from build123d import *

# Parameters (mm, degrees)
SKETCH1_R           = 4
BOSS_EXTRUDE1_DEPTH = 5
BOSS_EXTRUDE2_DEPTH = 29
FILLET1_R           = 50
FILLET2_R           = 50


with BuildPart() as part:
    # Sketch1 → Boss-Extrude1 (new body)
    with BuildSketch(Plane(origin=(0, 0, 0), x_dir=(1, 0, 0), z_dir=(0, 1, 0))):
        Polygon((-17.6, 10.161364738), (-17.6, 93), (17.6, 93), (17.6, 10.161364738), (89.340362552, -31.257952893), (71.740362552, -61.742047107), (0, -20.322729475), (-71.740362552, -61.742047107), (-89.340362552, -31.257952893), align=None)
        with Locations(Location((0, 0, 0), (0, 0, 270))):
            Circle(SKETCH1_R, mode=Mode.SUBTRACT)
        with BuildLine():
            Line((-11.5, 75), (-11.5, 71))
            ThreePointArc((-11.5, 71), (0, 59.5), (11.5, 71))
            Line((11.5, 71), (11.5, 75))
            ThreePointArc((11.5, 75), (0, 86.5), (-11.5, 75))
        make_face(mode=Mode.SUBTRACT)
        with BuildLine():
            Line((-14.875, 88), (-14.875, 84))
            ThreePointArc((-14.875, 84), (-13, 82.125), (-11.125, 84))
            Line((-11.125, 84), (-11.125, 88))
            ThreePointArc((-11.125, 88), (-13, 89.875), (-14.875, 88))
        make_face(mode=Mode.SUBTRACT)
        with BuildLine():
            Line((11.125, 88), (11.125, 84))
            ThreePointArc((11.125, 84), (13, 82.125), (14.875, 84))
            Line((14.875, 84), (14.875, 88))
            ThreePointArc((14.875, 88), (13, 89.875), (11.125, 88))
        make_face(mode=Mode.SUBTRACT)
        with BuildLine():
            Line((11.125, 62), (11.125, 58))
            ThreePointArc((11.125, 58), (13, 56.125), (14.875, 58))
            Line((14.875, 58), (14.875, 62))
            ThreePointArc((14.875, 62), (13, 63.875), (11.125, 62))
        make_face(mode=Mode.SUBTRACT)
        with BuildLine():
            Line((-14.875, 62), (-14.875, 58))
            ThreePointArc((-14.875, 58), (-13, 56.125), (-11.125, 58))
            Line((-11.125, 58), (-11.125, 62))
            ThreePointArc((-11.125, 62), (-13, 63.875), (-14.875, 62))
        make_face(mode=Mode.SUBTRACT)
    extrude(amount=BOSS_EXTRUDE1_DEPTH)

    # Sketch2 → Boss-Extrude2 (add)
    with BuildSketch(Plane.XZ):
        Polygon((-71.740362552, 61.742047107), (-89.340362552, 31.257952893), (-68.555752861, 19.257952893), (-50.955752861, 49.742047107), align=None)
        Polygon((71.740362552, 61.742047107), (89.340362552, 31.257952893), (68.555752861, 19.257952893), (50.955752861, 49.742047107), align=None)
    extrude(amount=BOSS_EXTRUDE2_DEPTH)

    # Fillet1
    # the kernel refuses this fillet: 50 mm, written as the material it adds along each edge
    with BuildSketch(Plane(origin=(-68.555752861, 0, 19.257952893), x_dir=(0, -1, 0), z_dir=(0.4999999999999999, 0, 0.8660254037844387))) as fillet1_piece_1:
        with BuildLine():
            CenterArc((50, 45.376205218), FILLET1_R, 180, 65.16541251)
            Line((0, 45.376205218), (-1, 45.376205218))
            Line((-1, 45.376205218), (-1, 0))
            Line((-1, 0), (0, -1))
            ThreePointArc((0, -1), (14.5, -1), (28.58, -0.907524104))
            Line((28.58, -0.907524104), (29, 0))
        make_face()
    extrude(amount=35.2)
    with BuildSketch(Plane(origin=(68.555752861, 0, 19.257952893), x_dir=(0, -1, 0), z_dir=(-0.49999999999999983, 0, 0.8660254037844388))) as fillet1_piece_2:
        with BuildLine():
            CenterArc((50, -45.376205218), FILLET1_R, 114.83458749, 65.16541251)
            Line((0, -45.376205218), (-1, -45.376205218))
            Line((-1, -45.376205218), (-1, 0))
            Line((-1, 0), (0, 1))
            ThreePointArc((0, 1), (14.5, 1), (28.58, 0.907524104))
            Line((28.58, 0.907524104), (29, 0))
        make_face()
    extrude(amount=35.2)
    # the kernel refuses this fillet: 50 mm, written as the material it takes off along each edge
    with BuildSketch(Plane(origin=(148.553958964, 5, -71.30300459), x_dir=(-0.8660254037844363, 0, -0.5000000000000039), z_dir=(-0.5000000000000039, 0, 0.8660254037844364)), Plane(origin=(-12.52676614, 5, 164.30300459), x_dir=(0.8660254037844429, 0, -0.4999999999999925), z_dir=(-0.49999999999999256, 0, -0.866025403784443))) as fillet1_2_piece_1:
        with BuildLine():
            CenterArc((47.370877129, 50), FILLET1_R, 198.662924885, 71.337075115)
            Line((0, 34), (-0.947417543, 33.68))
            ThreePointArc((-0.947417543, 33.68), (-1, 17), (-1, 0))
            Line((-1, 0), (0, -1))
            Line((0, -1), (47.370877129, -1))
            Line((47.370877129, -1), (47.370877129, 0))
        make_face()
    extrude(amount=272.054385647, mode=Mode.SUBTRACT)

    # Fillet2
    # the kernel refuses this fillet: 50 mm, written as the material it takes off along each edge
    with BuildSketch(Plane(origin=(-98.555752861, -29, -32.703571334), x_dir=(0.49710588531055566, 0.8188493868753551, -0.2870042166997965), z_dir=(0.4999999999999999, 0, 0.8660254037844387))) as fillet2_piece_1:
        with BuildLine():
            CenterArc((26.55146204, 49.210454923), FILLET2_R, 216.239467537, 43.564898237)
            Line((-13.776202402, 19.652385285), (-14.58275569, 19.061223892))
            ThreePointArc((-14.58275569, 19.061223892), (-7.706950588, 9.252184209), (-0.818849387, -0.574008433))
            Line((-0.818849387, -0.574008433), (0.177009747, -0.984209098))
            ThreePointArc((0.177009747, -0.984209098), (8.850487347, -0.210454923), (17.523964946, -0.984209098))
            Line((17.523964946, -0.984209098), (17.700974693, 0))
        make_face()
    extrude(amount=155.2, mode=Mode.SUBTRACT)
    with BuildSketch(Plane(origin=(98.555752861, -29, -32.703571334), x_dir=(-0.4971058853105562, 0.8188493868753546, -0.2870042166997967), z_dir=(-0.49999999999999983, 0, 0.8660254037844388))) as fillet2_piece_2:
        with BuildLine():
            CenterArc((26.55146204, -49.210454923), FILLET2_R, 100.195634226, 43.564898237)
            Line((-13.776202402, -19.652385285), (-14.58275569, -19.061223892))
            ThreePointArc((-14.58275569, -19.061223892), (-7.706950588, -9.252184209), (-0.818849387, 0.574008433))
            Line((-0.818849387, 0.574008433), (0.177009747, 0.984209098))
            ThreePointArc((0.177009747, 0.984209098), (8.850487347, 0.210454923), (17.523964946, 0.984209098))
            Line((17.523964946, 0.984209098), (17.700974693, 0))
        make_face()
    extrude(amount=155.2, mode=Mode.SUBTRACT)


solid = part.part
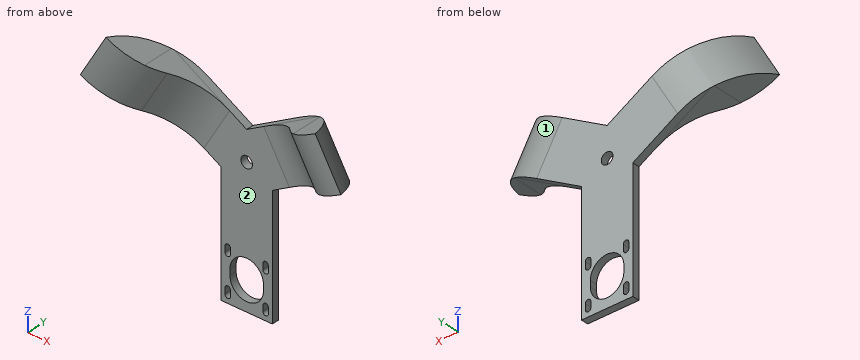
Model file for the job. Use its own axes, mm. Face numbers are marked on the shaded views. A direction names the side the tool comes from. Give positions to 0.01 mm unless a question says otherwise; leave off trailing zeros. Loops run counter-clockwise (first coordinate to the right, second up) from the corner with the lowest first, then second, coordinate; pieces in that order, holes last.
Item 1: Slice it at D-D (z = -31). Write the cut outline in (x, y).
Check values:
outline: (-17.6, 0) - (17.6, 0) - (17.6, 5) - (-17.6, 5) - close
Item 2: Slice it at A-A (z = -73). Write the cut outline in (x, y).
Check values:
outline: (-17.6, 0) - (-11.5, 0) - (-11.5, 5) - (-17.6, 5) - close; (11.5, 0) - (17.6, 0) - (17.6, 5) - (11.5, 5) - close
Item 3: Which spindle directions (+Z, -Z, +X, -X, +Y, -Y) get a long thin tool onto all of the face, cutting with end or side? Do the marked faces 1 and 2. Say none if no direction does.
Check values:
face 1: +Z, +X, +Y
face 2: -Z, -Y
Item 4: Drill centre lines: line 1 along X through (y, z) = (2.6, 0); line 2 along X through (y, z) = (-18, 49); line 3 along Y through (x, z) = (53, 37). Where is each one in solid material? Low to high.
Check values:
line 1: x = -35.2 to -4, 4 to 35.2
line 2: x = -72.99 to -49.67, 49.67 to 72.99
line 3: y = -19.27 to 1.34
Item 5: Slice it at C-C (x = 6). Write the cut outline in (y, z).
Check values:
outline: (0, -93) - (5, -93) - (5, -84.81) - (0, -84.81) - close; (0, -61.19) - (5, -61.19) - (5, 23.79) - (0, 23.79) - close
Item 6: Drop flat-ended pins along their axis: P1, Ø2, axis at y = 2.5, z = -60, coming from the -X side; P2, Ø4.5, axis at y = 3, z = -73, coming from the +X side; P3, Ø9, axis at x = 0, z = 0, coming from the -Y side. Give the stop position or say it passes through.
Check values:
P1: stops at x = -17.6
P2: stops at x = 17.6
P3: stops at y = 0
Item 7: Slice it at B-B (y = -4). Write the cut outline in (x, z).
Check values:
outline: (-73.1, 21.88) - (-46.23, 6.37) - (-28.63, 36.85) - (-55.5, 52.37) - close; (28.63, 36.85) - (46.23, 6.37) - (73.1, 21.88) - (55.5, 52.37) - close
